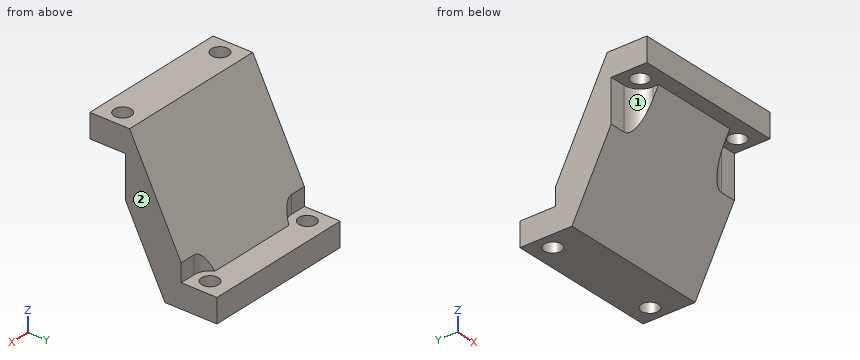
```python
from build123d import *

# Parameters (mm, degrees)
BOSS_EXTRUDE1_DEPTH     = 19
CUT_EXTRUDE1_DEPTH      = 48.801673611
CUT_EXTRUDE1_DEPTH_BACK = 48.801673611
SKETCH5_R               = 2.15
SKETCH6_R               = 2.15
CUT_EXTRUDE2_DEPTH      = 6
CUT_EXTRUDE6_DEPTH      = 48.801673611
CUT_EXTRUDE7_DEPTH      = 36


with BuildPart() as part:
    # Sketch2 → Boss-Extrude1 (new, symmetric)
    with BuildSketch(Plane(origin=(0, 0, 0), x_dir=(0, 0, -1), z_dir=(1, 0, 0))):
        Polygon((0, 0), (6, 0), (6, 3.6), (36, 18.885763485), (36, 32), (30, 32), (30, 25.285763485), (0, 10), align=None)
    extrude(amount=BOSS_EXTRUDE1_DEPTH, both=True)

    # Sketch5 → Cut-Extrude1 (cut, two sides: drawn at the far end of the back side and taken through both)
    with BuildSketch(Plane.XY.offset(-30).offset(-CUT_EXTRUDE1_DEPTH_BACK)):
        with Locations((-15, 27)):
            Circle(SKETCH5_R)
        with Locations(Location((15, 27, 0), (0, 0, 307.125127623))):
            Circle(SKETCH5_R)
    extrude(amount=CUT_EXTRUDE1_DEPTH + CUT_EXTRUDE1_DEPTH_BACK, mode=Mode.SUBTRACT)

    # Sketch6 → Cut-Extrude2 (cut)
    with BuildSketch(Plane.XY):
        with Locations((-15, 5)):
            Circle(SKETCH6_R)
        with Locations(Location((15, 5, 0), (0, 0, 319.370671217))):
            Circle(SKETCH6_R)
    extrude(amount=-CUT_EXTRUDE2_DEPTH, mode=Mode.SUBTRACT)

    # Sketch9 → Cut-Extrude6 (cut, through all)
    with BuildSketch(Plane(origin=(0, 0, -6), x_dir=(-1, 0, 0), z_dir=(0, 0, -1))):
        with BuildLine():
            Line((-19, 0), (-19, 9))
            Line((-19, 9), (-15, 9))
            ThreePointArc((-15, 9), (-12.171572875, 7.828427125), (-11, 5))
            Line((-11, 5), (-11, 0))
            Line((-11, 0), (-19, 0))
        make_face()
        with BuildLine():
            Line((19, 0), (19, 9))
            Line((19, 9), (15, 9))
            ThreePointArc((15, 9), (12.171572875, 7.828427125), (11, 5))
            Line((11, 5), (11, 0))
            Line((11, 0), (19, 0))
        make_face()
    extrude(amount=CUT_EXTRUDE6_DEPTH, mode=Mode.SUBTRACT)

    # Sketch11 → Cut-Extrude7 (cut)
    with BuildSketch(Plane.XY.offset(-30)):
        with BuildLine():
            Line((11, 32), (19, 32))
            Line((19, 32), (19, 23))
            Line((19, 23), (15, 23))
            ThreePointArc((15, 23), (12.171572875, 24.171572875), (11, 27))
            Line((11, 27), (11, 32))
        make_face()
        with BuildLine():
            Line((-19, 23), (-15, 23))
            ThreePointArc((-15, 23), (-12.171572875, 24.171572875), (-11, 27))
            Line((-11, 27), (-11, 32))
            Line((-11, 32), (-19, 32))
            Line((-19, 32), (-19, 23))
        make_face()
    extrude(amount=CUT_EXTRUDE7_DEPTH, mode=Mode.SUBTRACT)


solid = part.part
```
Geometry check sheet. Reference: the model listing, model coordinates, mm. Face numbers are marked on the shaded views. A direction names the side the tool comes from. Coordinates: 2 decimals unless noted, no trailing zeros. Order: outer loops, then holes, each group sorted by start corner. A loop starts at its lowest first (then second) coordinate and runs counter-clockwise, first axis right, second up. Notation, with made-up numbers: (87.25, 4) - (101.25, 4) arc R14 ccw to (101.25, 9) - close; hole circle Ø3 at (1, -29). An arc over 180 degrees is marked (long way). Answer in a Markdown table with one row per item. Add a question column.
1. Access from +Z, -Z, +X, -X, +Y, -Y to the whole of each face (thin tool, end or side, straight path). Record for the marked faces 1 and 2.
2. Section check D-D (y = 2). Enter the section's corners in (x, z), plus the area to 3 significant figures.
3. Section check A-A (y = 27). Enter the section's corners in (x, z), plus the area to 3 significant figures.
4. Gauge pin test, flat ends, axial feed: pin 1 Ø4.5 at (x, z) = (16.5, -29) entering from +Y; pin 2 Ø5.5 at (x, y) = (-15, 27) entering from +Z; pin 3 Ø1 at (x, z) = (2, -6) entering from +Y; pin 4 Ø2 at (x, z) = (-17.5, -9.5) entering from -Y. Record the tip position at first contact, or that the pin passes through.
5. Section check B-B (x = -16). Enter the section's corners in (y, z), plus the area to 3 significant figures.
6. Material ranges on L1, parallel to X at y = 27, z = -33.25; L2, parallel to Z at x = 4, y = 2; L3, parallel to Z at x = -7, y = 28.5, recorded low to high. Write a range as [from, to].
7. Section check C-C (x = -3). Enter the section's corners in (y, z).
Data:
| question | item | result |
|---|---|---|
| 1 | face 1 | -Z, -X, -Y |
| 1 | face 2 | +Z, -Z, +X, +Y, -Y |
| 2 | outline | (-19, -6) - (19, -6) - (19, 0) - (-19, 0) - close |
| 2 | area | 228 mm² |
| 3 | outline | (-19, -36) - (-17.15, -36) - (-17.15, -30) - (-19, -30) - close; (-12.85, -36) - (12.85, -36) - (12.85, -30) - (-12.85, -30) - close; (17.15, -36) - (19, -36) - (19, -30) - (17.15, -30) - close |
| 3 | area | 176 mm² |
| 4 | pin 1 | stops at y = 32 |
| 4 | pin 2 | stops at z = -30 |
| 4 | pin 3 | stops at y = 13.31 |
| 4 | pin 4 | stops at y = 9 |
| 5 | outline | (0, -6) - (3.1, -6) - (3.1, 0) - (0, 0) - close; (6.9, -6) - (9, -6) - (9, -16.6) - (18.89, -36) - (25.1, -36) - (25.1, -30) - (23, -30) - (23, -25.51) - (10, 0) - (6.9, 0) - close; (28.9, -36) - (32, -36) - (32, -30) - (28.9, -30) - close |
| 5 | area | 305 mm² |
| 6 | L1 | x = [-19, -17.15], [-12.85, 12.85], [17.15, 19] |
| 6 | L2 | z = [-6, 0] |
| 6 | L3 | z = [-36, -30] |
| 7 | outline | (0, -6) - (3.6, -6) - (18.89, -36) - (32, -36) - (32, -30) - (25.29, -30) - (10, 0) - (0, 0) - close |
